from build123d import *

# Parameters (mm, degrees)
SKETCH_1_R          = 5.03
SKETCH_1_R_2        = 1.5
SKETCH_1_W          = 8.5
SKETCH_1_H          = 4.5
EXTRUDE_1_DEPTH     = 4
SKETCH_2_R          = 6
EXTRUDE_2_DEPTH     = 4
SKETCH_3_R          = 2
CUT_EXTRUDE_1_DEPTH = 4


with BuildPart() as part:
    # 草图1 → 凸台-拉伸1 (new body)
    with BuildSketch(Plane.XY):
        with BuildLine():
            Line((87, -4.5), (9.367496998, -4.5))
            ThreePointArc((9.367496998, -4.5), (8.068458892, -4.795836543), (7.025622748, -5.625))
            ThreePointArc((7.025622748, -5.625), (-7.794228634, -4.5), (-1.358581522, 8.896867777))
            ThreePointArc((-1.358581522, 8.896867777), (-0.119086833, 9.385408641), (0.786634182, 10.36249037))
            Line((0.786634182, 10.36249037), (13.919137184, 33.108652801))
            ThreePointArc((13.919137184, 33.108652801), (14.312454275, 34.381571072), (14.11579573, 35.699275393))
            ThreePointArc((14.11579573, 35.699275393), (20.177098522, 47.666206639), (31.398879943, 40.316481698))
            ThreePointArc((31.398879943, 40.316481698), (31.879352208, 39.085435776), (32.842164256, 38.180272466))
            Line((32.842164256, 38.180272466), (87.068435314, 6.227425402))
            ThreePointArc((87.068435314, 6.227425402), (87.55756519, 6.02099445), (88.083774649, 5.950529007))
            Line((88.083774649, 5.950529007), (96, 5.950529007))
            ThreePointArc((96, 5.950529007), (97.414213562, 5.364742569), (98, 3.950529007))
            Line((98, 3.950529007), (98, 0))
            Line((98, 0), (98, -2.5))
            ThreePointArc((98, -2.5), (97.414213562, -3.914213562), (96, -4.5))
            Line((96, -4.5), (87, -4.5))
        make_face()
        Circle(SKETCH_1_R, mode=Mode.SUBTRACT)
        with Locations((22.5, 38.97114317)):
            Circle(SKETCH_1_R, mode=Mode.SUBTRACT)
        with Locations((30, 0)):
            Circle(SKETCH_1_R_2, mode=Mode.SUBTRACT)
        with Locations((60, 0)):
            Circle(SKETCH_1_R_2, mode=Mode.SUBTRACT)
        with Locations((45, 0)):
            Rectangle(SKETCH_1_W, SKETCH_1_H, mode=Mode.SUBTRACT)
        with BuildLine():
            Line((21.255373367, 27.815386605), (12.124355653, 12))
            ThreePointArc((12.124355653, 12), (12.124355653, 7), (16.454482672, 4.5))
            Line((16.454482672, 4.5), (58.367468971, 4.5))
            ThreePointArc((58.367468971, 4.5), (63.210197148, 8.25582003), (60.777559131, 13.880806481))
            Line((60.777559131, 13.880806481), (30.521886072, 30.525892321))
            ThreePointArc((30.521886072, 30.525892321), (28.338019103, 31.139965525), (26.107583087, 30.725820601))
            ThreePointArc((26.107583087, 30.725820601), (25.308251431, 30.420486827), (24.483535962, 30.192442521))
            ThreePointArc((24.483535962, 30.192442521), (22.620790776, 29.341612745), (21.255373367, 27.815386605))
        make_face(mode=Mode.SUBTRACT)
        with Locations((75, 0)):
            Rectangle(SKETCH_1_W, SKETCH_1_H, mode=Mode.SUBTRACT)
    extrude(amount=EXTRUDE_1_DEPTH)

    # 草图2 → 凸台-拉伸2 (add)
    with BuildSketch(Plane.XY.offset(4)):
        with Locations((39.819566523, 34.068836013)):
            Circle(SKETCH_2_R)
    extrude(amount=-EXTRUDE_2_DEPTH)

    # 草图3 → 切除-拉伸1 (cut)
    with BuildSketch(Plane.XY.offset(4)):
        with Locations((39.819566523, 34.068836013)):
            Circle(SKETCH_3_R)
    extrude(amount=-CUT_EXTRUDE_1_DEPTH, mode=Mode.SUBTRACT)


solid = part.part
Geometry check sheet. Reference: the model listing, model coordinates, mm. A direction names the side the tool comes from. Give positions to 0.01 mm unless a question says otherwise; leave off trailing zeros. Loops run counter-clockwise (first coordinate to the right, second up) from the corner with the lowest first, then second, coordinate; pieces in that order, holes last. Notation, with made-up numbers: M 78,10.25 L 95,10.25 A24 cw 95,44.25 Z; hole C 66,-36.5 d8. An arc over 180 degrees is marked long. Answer as a JSON object with one key per item and string values. Group by question number.
Item 1: Sectioned sample at A-A on x = 39. Record the boundary of the cut face in (y, z), plus the area to 3 significant figures.
Item 2: Sectioned sample at D-D on y = 41.5. Record the boundary of the cut face in (x, z).
Item 3: Mould release check, pull along Y, two halves, no side actions. Record for faces 1 (the flat face through (44, 24, 0)), 2 (the flat face through (79.25, 0, 2)), 3 (the cylindrical face through (-7.67, -4.71, 1.97)): pulls with the +Y half, pulls with the -Y half, needs draft (parallel to the pull), parting line crosses it, or undercut.
Item 4: Access from +Z, -Z, +X, -X, +Y, -Y to the whole of each face (thin tool, end or side, straight path). Record for faces 4 (the flat face through (53, -4.5, 2)), 5 (the flat face through (98, 1, 2)), 6 (the cylindrical face through (22.644, 29.359, 1.972)).
Item 5: Gauge pin test, flat ends, axial feed: pin 1 (2 mm diameter, centred on x = 80, z = 1.5, fed in from +Y); pin 2 (2 mm diameter, centred on x = 43.5, z = 2.5, fed in from -Y); pin 3 (2 mm diameter, centred on y = 23, z = 1.5, fed in from -X). Record the tip position at first contact, or that the pin passes through.
Item 6: Sectioned sample at C-C on x = 2. Record the boundary of the cut face in (y, z), plus the area to 3 significant figures.
Item 7: Sectioned sample at B-B on y = 0. Record the boundary of the cut face in (x, z), plus the area to 3 significant figures.
Item 8: Material ranges on L1, parallel to X at y = 39.5, z = 0.6; L2, parallel to Y at x = 49, z = 2.2; L3, parallel to Y at x = 60, z = 0.9, recorded low to high.
Findings below:
{
 "1": {"outline": "M -4.5,0 L 4.5,0 L 4.5,4 L -4.5,4 Z; M 25.86,0 L 32.24,0 L 32.24,4 L 25.86,4 Z; M 35.89,0 L 40.01,0 L 40.01,4 L 35.89,4 Z", "area": "78.0 mm2"},
 "2": {"outline": "M 13.86,0 L 18.15,0 L 18.15,4 L 13.86,4 Z; M 26.85,0 L 31.14,0 L 31.14,4 L 26.85,4 Z"},
 "3": {"face 1": "needs draft", "face 2": "undercut", "face 3": "parting line crosses it"},
 "4": {"face 4": "+Z, -Z, +X, -Y", "face 5": "+Z, -Z, +X, +Y, -Y", "face 6": "+Z, -Z"},
 "5": {"pin 1": "y = 10.98", "pin 2": "y = -4.5", "pin 3": "x = 7.51"},
 "6": {"outline": "M -8.77,0 L -4.62,0 L -4.62,4 L -8.77,4 Z; M 4.62,0 L 12.46,0 L 12.46,4 L 4.62,4 Z", "area": "48.0 mm2"},
 "7": {"outline": "M -9,0 L -5.03,0 L -5.03,4 L -9,4 Z; M 5.03,0 L 28.5,0 L 28.5,4 L 5.03,4 Z; M 31.5,0 L 40.75,0 L 40.75,4 L 31.5,4 Z; M 49.25,0 L 58.5,0 L 58.5,4 L 49.25,4 Z; M 61.5,0 L 70.75,0 L 70.75,4 L 61.5,4 Z; M 79.25,0 L 98,0 L 98,4 L 79.25,4 Z", "area": "296 mm2"},
 "8": {"L1": "13.52 to 17.5, 27.5 to 31.64, 37.27 to 42.37", "L2": "-4.5 to -2.25, 2.25 to 4.5, 20.36 to 28.66", "L3": "-4.5 to -1.5, 1.5 to 4.77, 14.31 to 22.18"}
}
